Can you work these out from the model? Positions are in its coordinate system, mm. Coordinates: 2 decimals unless noted, no trailing zeros. Write each loop counter-clockwise with the first axis right and the second up, starting at its lowest first coordinate (ties: lowest second). Pieces come first, ordered by that corner, then holes. Notation, with made-up numbers: M 1.5,-3.75 L 22.5,-3.75 A26 ccw 22.5,19.25 Z; hole C -7.75,-2.75 d11. An arc over 180 degrees is marked long. Answer as a JSON object with one key per item and string values. Group by question number.
from build123d import *

# Parameters (mm, degrees)
BOSS_EXTRUDE1_DEPTH      = 1.5
M3_CLEARANCE_HOLE1_D     = 3.2
M3_CLEARANCE_HOLE1_DEPTH = 3
SKETCH5_R                = 15
CUT_EXTRUDE1_DEPTH       = 1
CUT_EXTRUDE1_DEPTH_BACK  = 4


with BuildPart() as part:
    # Sketch1 → Boss-Extrude1 (new body, symmetric)
    with BuildSketch(Plane(origin=(0, 0, 0), x_dir=(1, 0, 0), z_dir=(0, 1, 0))):
        with BuildLine():
            Line((50, 10), (84, 10))
            ThreePointArc((84, 10), (88.242640687, 8.242640687), (90, 4))
            Line((90, 4), (90, -4))
            ThreePointArc((90, -4), (88.242640687, -8.242640687), (84, -10))
            Line((84, -10), (50, -10))
            ThreePointArc((50, -10), (21.715728753, -21.715728753), (10, -50))
            Line((10, -50), (10, -84))
            ThreePointArc((10, -84), (8.242640687, -88.242640687), (4, -90))
            Line((4, -90), (-4, -90))
            ThreePointArc((-4, -90), (-8.242640687, -88.242640687), (-10, -84))
            Line((-10, -84), (-10, -50))
            ThreePointArc((-10, -50), (-21.715728753, -21.715728753), (-50, -10))
            Line((-50, -10), (-84, -10))
            ThreePointArc((-84, -10), (-88.242640687, -8.242640687), (-90, -4))
            Line((-90, -4), (-90, 4))
            ThreePointArc((-90, 4), (-88.242640687, 8.242640687), (-84, 10))
            Line((-84, 10), (-50, 10))
            ThreePointArc((-50, 10), (-21.715728753, 21.715728753), (-10, 50))
            Line((-10, 50), (-10, 84))
            ThreePointArc((-10, 84), (-8.242640687, 88.242640687), (-4, 90))
            Line((-4, 90), (4, 90))
            ThreePointArc((4, 90), (8.242640687, 88.242640687), (10, 84))
            Line((10, 84), (10, 50))
            ThreePointArc((10, 50), (21.715728753, 21.715728753), (50, 10))
        make_face()
    extrude(amount=BOSS_EXTRUDE1_DEPTH, both=True)

    # M3 Clearance Hole1
    with Locations(Plane(origin=(0, 1.5, 0), x_dir=(1, 0, 0), z_dir=(0, 1, 0))):
        with Locations((-84, 4), (-84, -4), (-4, 84), (4, 84), (84, 4), (84, -4), (4, -84), (-4, -84), (-39, 4), (-39, -4), (39, 4), (39, -4), (4, -39), (-4, -39), (-4, 39), (4, 39)):
            Hole(M3_CLEARANCE_HOLE1_D / 2, depth=M3_CLEARANCE_HOLE1_DEPTH)

    # Sketch5 → Cut-Extrude1 (cut, two sides)
    with BuildSketch(Plane(origin=(0, 1.5, 0), x_dir=(1, 0, 0), z_dir=(0, 1, 0))) as cut_extrude1_sk:
        Circle(SKETCH5_R)
    extrude(amount=CUT_EXTRUDE1_DEPTH, mode=Mode.SUBTRACT)
    extrude(cut_extrude1_sk.sketch, amount=-CUT_EXTRUDE1_DEPTH_BACK, mode=Mode.SUBTRACT)


solid = part.part
Q1. If we section it at A-A on z = 0: List the corners of the cut face in (x, y) for me.
Q2. Please list where these lines run through material, in increasing order: L1, parallel to Z at x = -39, y = -0.4; L2, parallel to X at y = -0.8, z = 84; L3, parallel to Z at x = 4, y = -0.25.
Q3. If we section it at D-D on x = -61: List the corners of the cut face in (y, z) for me, and give its area (3 significant figures).
Q4. If we section it at B-B on y = 0.95: Give the number of separate pieces and of enclosed holes in the cut face, and give its area (3 significant figures).
Q5. If we section it at C-C on z = -69: List the corners of the cut face in (x, y) for me.
Q6. Will these pins go through, and if not, where does the flat tip stop? pin 1 (1.5 mm diameter, centred on x = -24, y = -1, fed in from -Z); pin 2 (1.5 mm diameter, centred on x = 64, y = 0.5, fed in from +Z); pin 3 (1 mm diameter, centred on y = -1, z = -57.5, fed in from -X).
Q7. We'd pull the mould along Z, two halves only. Please class faces 1 (the cylindrical face through (8.196, 0.021, -88.289)), 2 (the cylindrical face through (88.289, 0.021, 8.196)), 3 (the cylindrical face through (-14.985, 0.021, -0.66)): pulls with the +Z half, pulls with the -Z half, needs draft (parallel to the pull), parting line crosses it, or undercut.
Reply:
{
 "1": {"outline": "M -90,-1.5 L -15,-1.5 L -15,1.5 L -90,1.5 Z; M 15,-1.5 L 90,-1.5 L 90,1.5 L 15,1.5 Z"},
 "2": {"L1": "-11.54 to -5.6, -2.4 to 2.4, 5.6 to 11.54", "L2": "-10 to -5.6, -2.4 to 2.4, 5.6 to 10", "L3": "-90 to -85.6, -82.4 to -40.6, -37.4 to -14.46, 14.46 to 37.4, 40.6 to 82.4, 85.6 to 90"},
 "3": {"outline": "M -1.5,-10 L 1.5,-10 L 1.5,10 L -1.5,10 Z", "area": "60.0 mm^2"},
 "4": {"separate pieces": "1", "enclosed holes": "17", "area": "7,280 mm^2"},
 "5": {"outline": "M -10,-1.5 L 10,-1.5 L 10,1.5 L -10,1.5 Z"},
 "6": {"pin 1": "z = -20.26", "pin 2": "z = 10", "pin 3": "x = -10"},
 "7": {"face 1": "pulls with the -Z half", "face 2": "pulls with the +Z half", "face 3": "undercut"}
}
